Build history of the part. All positions in model axes, mm. A direction names the side the tool comes from. Give positions to 0.01 mm unless a question says otherwise; leave off trailing zeros. Order: outer loops, then holes, each group sorted by start corner. A loop starts at its lowest first (then second) coordinate and runs counter-clockwise, first axis right, second up. Notation, with made-up numbers: M 58.25,84 L 86.25,84 A26 ccw 86.25,115 Z; hole C 45.5,54.5 d11. An arc over 180 degrees is marked long. One line per item, written item: value. Start each with the question number.
from build123d import *

# Parameters (mm, degrees)
SKETCH2_W           = 82.55
SKETCH2_H           = 31.75
SKETCH2_W_2         = 76.2
SKETCH2_H_2         = 25.4
EXTRUDE_THIN1_DEPTH = 508
BOSS_EXTRUDE2_DEPTH = 31.75
BOSS_EXTRUDE3_DEPTH = 3.175
BOSS_EXTRUDE4_DEPTH = 3.175
SKETCH6_R           = 6.35
SHAFT_HOLE_DEPTH    = 31.75
SKETCH7_W           = 3.175
SKETCH7_H           = 7.9375
KEYWAY_DEPTH        = 31.75
CUT_EXTRUDE1_START  = -76.651281
SKETCH8_R           = 6.35
CUT_EXTRUDE1_DEPTH  = 57.601281
BOSS_EXTRUDE5_DEPTH = 3.175
BOSS_EXTRUDE6_DEPTH = 3.175
CUT_EXTRUDE2_START  = -82.55
SKETCH11_R          = 3.175
CUT_EXTRUDE2_DEPTH  = 82.55
CUT_EXTRUDE3_START  = -31.75
SKETCH12_W          = 76.2
SKETCH12_H          = 254
CUT_EXTRUDE3_DEPTH  = 31.75


with BuildPart() as part:
    # Sketch2 → Extrude-Thin1 (new body)
    with BuildSketch(Plane(origin=(0, 0, 0), x_dir=(1, 0, 0), z_dir=(0, 1, 0))):
        with Locations((22.913756614, 0.671957672)):
            Rectangle(SKETCH2_W, SKETCH2_H)
        with Locations((22.913756614, 0.671957672)):
            Rectangle(SKETCH2_W_2, SKETCH2_H_2, mode=Mode.SUBTRACT)
    extrude(amount=EXTRUDE_THIN1_DEPTH)

    # Sketch3 → Boss-Extrude2 (add)
    with BuildSketch(Plane(origin=(0, 0, -16.546957672), x_dir=(-1, 0, 0), z_dir=(0, 0, -1))):
        with BuildLine():
            Line((-64.188756614, 0), (-48.313756614, 0))
            ThreePointArc((-48.313756614, 0), (-22.913756614, -25.4), (2.486243386, 0))
            Line((2.486243386, 0), (18.361243386, 0))
            ThreePointArc((18.361243386, 0), (-22.913756614, -41.275), (-64.188756614, 0))
        make_face()
    extrude(amount=-BOSS_EXTRUDE2_DEPTH)

    # Sketch4 → Boss-Extrude3 (add)
    with BuildSketch(Plane(origin=(0, 0, -16.546957672), x_dir=(-1, 0, 0), z_dir=(0, 0, -1))):
        with BuildLine():
            Line((-48.313756614, 0), (2.486243386, 0))
            ThreePointArc((2.486243386, 0), (-22.913756614, -25.4), (-48.313756614, 0))
        make_face()
    extrude(amount=-BOSS_EXTRUDE3_DEPTH)

    # Sketch5 → Boss-Extrude4 (add)
    with BuildSketch(Plane.XY.offset(15.203042328)):
        with BuildLine():
            Line((-2.486243386, 0), (48.313756614, 0))
            ThreePointArc((48.313756614, 0), (22.913756614, -25.4), (-2.486243386, 0))
        make_face()
    extrude(amount=-BOSS_EXTRUDE4_DEPTH)

    # Sketch6 → Shaft Hole (cut)
    with BuildSketch(Plane(origin=(0, 0, -16.546957672), x_dir=(-1, 0, 0), z_dir=(0, 0, -1))):
        with Locations((-22.913756614, 0)):
            Circle(SKETCH6_R)
    extrude(amount=-SHAFT_HOLE_DEPTH, mode=Mode.SUBTRACT)

    # Sketch7 → Keyway (cut)
    with BuildSketch(Plane(origin=(0, 0, -16.546957672), x_dir=(-1, 0, 0), z_dir=(0, 0, -1))):
        with Locations((-22.913756614, 3.96875)):
            Rectangle(SKETCH7_W, SKETCH7_H)
    extrude(amount=-KEYWAY_DEPTH, mode=Mode.SUBTRACT)

    # Sketch8 → Cut-Extrude1 (cut)
    with BuildSketch(Plane(origin=(0, 262.273478836, -262.273478836), x_dir=(-1, 0, 0), z_dir=(0, 0.707106781, -0.707106781)).offset(CUT_EXTRUDE1_START)):
        with Locations((-22.913756614, 322.109778865)):
            Circle(SKETCH8_R)
    extrude(amount=CUT_EXTRUDE1_DEPTH, mode=Mode.SUBTRACT)

    # Sketch9 → Boss-Extrude5 (add)
    with BuildSketch(Plane.ZY.offset(18.361243386)):
        with BuildLine():
            Line((-16.546957672, 508), (-3.846957672, 508))
            Line((-3.846957672, 508), (2.503042328, 508))
            Line((2.503042328, 508), (15.203042328, 508))
            ThreePointArc((15.203042328, 508), (-0.671957672, 523.875), (-16.546957672, 508))
        make_face()
    extrude(amount=-BOSS_EXTRUDE5_DEPTH)

    # Sketch10 → Boss-Extrude6 (add)
    with BuildSketch(Plane(origin=(64.188756614, 0, 0), x_dir=(0, 0, -1), z_dir=(1, 0, 0))):
        with BuildLine():
            Line((-12.028042328, 508), (13.371957672, 508))
            Line((13.371957672, 508), (16.546957672, 508))
            ThreePointArc((16.546957672, 508), (0.671957672, 523.875), (-15.203042328, 508))
            Line((-15.203042328, 508), (-12.028042328, 508))
        make_face()
    extrude(amount=-BOSS_EXTRUDE6_DEPTH)

    # Sketch11 → Cut-Extrude2 (cut)
    with BuildSketch(Plane.ZY.offset(18.361243386).offset(CUT_EXTRUDE2_START)):
        with Locations((-0.671957672, 508)):
            Circle(SKETCH11_R)
    extrude(amount=CUT_EXTRUDE2_DEPTH, mode=Mode.SUBTRACT)

    # Sketch12 → Cut-Extrude3 (cut)
    with BuildSketch(Plane(origin=(0, 0, -16.546957672), x_dir=(-1, 0, 0), z_dir=(0, 0, -1)).offset(CUT_EXTRUDE3_START)):
        with Locations((-22.913756614, 381)):
            Rectangle(SKETCH12_W, SKETCH12_H)
    extrude(amount=CUT_EXTRUDE3_DEPTH, mode=Mode.SUBTRACT)


solid = part.part
1) Slice it at B-B (y = 381.5). List the corners of the cut face in (x, z), plus the area to 3 significant figures.
2) Drop flat-ended pins along their axis: P1, Ø3.5, axis at x = 8, z = -14, coming from the +Y side; P2, Ø10, axis at x = 52, z = -6.5, coming from the +Y side. Give the stop position or say it passes through.
3) Tool access for faces 1 (the cylindrical face through (62.62, 523.87, -1.02)), 2 (the cylindrical face through (23.472, -25.394, -0.85)): list every direction of +Z, -Z, +X, -X, +Y, -Y with a clear straight run to the whole face (end or side of a thin tool).
4) Drill centre lines: line 1 (X direction, y = 287, z = -8.5); line 2 (Z direction, x = -17, y = 508); line 3 (Z direction, x = 23.5, y = 78.5). Where is each one in solid material? Low to high.
5) Slice it at A-A (y = 62). List the corners of the cut face in (x, z), plus the area to 3 significant figures.
6) Pull direction Z, two halves, no side cores. Call faces 3 (the flat face through (-15.186, 258, 0)), 4 (the flat face through (-18.361, 266, -1)), 5 (the cylindrical face through (-16.8, 523.87, -0.32)): pulls with the +Z half, pulls with the -Z half, needs draft (parallel to the pull), parting line crosses it, or undercut.
Results list:
1. outline: M -18.36,-16.55 L -15.19,-16.55 L -15.19,15.2 L -18.36,15.2 Z; M 61.01,-16.55 L 64.19,-16.55 L 64.19,15.2 L 61.01,15.2 Z
1. area: 202 mm²
2. P1: stops at y = 254
2. P2: stops at y = 0
3. face 1: +X, -X, +Y
3. face 2: +Y
4. line 1: x = -18.36 to -15.19, 61.01 to 64.19
4. line 2: z = -16.55 to -3.85, 2.5 to 15.2
4. line 3: z = -16.55 to -13.37, 12.03 to 15.2
5. outline: M -18.36,-16.55 L 64.19,-16.55 L 64.19,15.2 L -18.36,15.2 Z; hole M -15.19,-13.37 L 61.01,-13.37 L 61.01,12.03 L -15.19,12.03 Z
5. area: 685 mm²
6. face 3: undercut
6. face 4: needs draft
6. face 5: parting line crosses it
